Here's how the part is built. I have some questions about the finished solid (model axes, mm). A direction names the side the tool comes from. Give positions to 0.01 mm unless a question says otherwise; leave off trailing zeros. Loops run counter-clockwise (first coordinate to the right, second up) from the corner with the lowest first, then second, coordinate; pieces in that order, holes last.
Q1. I need wall thicknesses on line 1 (Y direction, x = 0.25, z = 1); line 2 (Z direction, x = 3, y = -2.75); line 3 (X direction, y = -1.25, z = 4.75). Which ranges of each line are inside material? Lowest first, please.
Q2. For faces 1 (the face through (-1.08, -4.88, 10.46)), 2 (the face through (0, 0, 0)), which set-ups out of +Z, -Z, +X, -X, +Y, -Y let a thin tool reach every point of the face, with its end or its side?
Q3. If we section it at C-C (z = 8.75): Please give me the cut outline in (x, y), plus the area to 3 significant figures.
Q4. Will these pins go through, and if not, where does the flat tip stop? P1, Ø1.5, axis at x = -0.5, z = 11, coming from the -Y side; P2, Ø4, axis at y = 5, z = 12.5, coming from the -X side; P3, Ø5, axis at y = -4.5, z = 10, coming from the -X side; P4, Ø4, axis at x = -0.5, z = 6.5, coming from the +Y side.
Q5. If we section it at D-D (z = 2.75): Please give me the cut outline in (x, y), plus the area to 3 significant figures.
from build123d import *

# Parameters (mm, degrees)
SKETCH1_R           = 7
BOSS_EXTRUDE1_DEPTH = 7
FILLET1_R           = 1
SKETCH2_R           = 5
BOSS_EXTRUDE2_DEPTH = 7
FILLET2_R           = 1


with BuildPart() as part:
    # Sketch1 → Boss-Extrude1 (new body)
    with BuildSketch(Plane.XY):
        Circle(SKETCH1_R)
    extrude(amount=BOSS_EXTRUDE1_DEPTH)

    # Fillet1
    fillet1_edges = [part.edges().sort_by_distance(p)[0] for p in [
        (-7, 0, 0),
        (-7, 0, 7),
    ]]
    fillet(fillet1_edges, radius=FILLET1_R)

    # Sketch2 → Boss-Extrude2 (add)
    with BuildSketch(Plane.XY.offset(7)):
        Circle(SKETCH2_R)
    extrude(amount=BOSS_EXTRUDE2_DEPTH)

    # Fillet2
    fillet2_edges = [part.edges().sort_by_distance(p)[0] for p in [
        (-5, 0, 7),
        (-5, 0, 14),
    ]]
    fillet(fillet2_edges, radius=FILLET2_R - 0.0001)  # a hair under: the kernel refuses the full size


solid = part.part
Check sheet entries:
1. line 1: y = -7 to 7
1. line 2: z = 0 to 14
1. line 3: x = -6.89 to 6.89
2. face 1: +Z
2. face 2: -Z, +X, -X, +Y, -Y
3. outline: circle Ø10 at (0, 0)
3. area: 78.5 mm2
4. P1: stops at y = -5
4. P2: stops at x = -4
4. P3: stops at x = -4.58
4. P4: stops at y = 7
5. outline: circle Ø14 at (0, 0)
5. area: 154 mm2
